Drawing for the job (mm, zero at the part's lowest x, y, z). A direction names the side the tool comes from. Coordinates: 2 decimals unless noted, no trailing zeros. Loops run counter-clockwise (first coordinate to the right, second up) from the corner with the lowest first, then second, coordinate; pieces in that order, holes last. Notation, with made-up numbers: (31.5, 75.5) - (83.5, 75.5) arc R15 cw to (83.5, 87.5) - close; hole circle Ø3 at (74, 6). An arc over 180 degrees is marked (long way). Put each result on its own line as item: value.
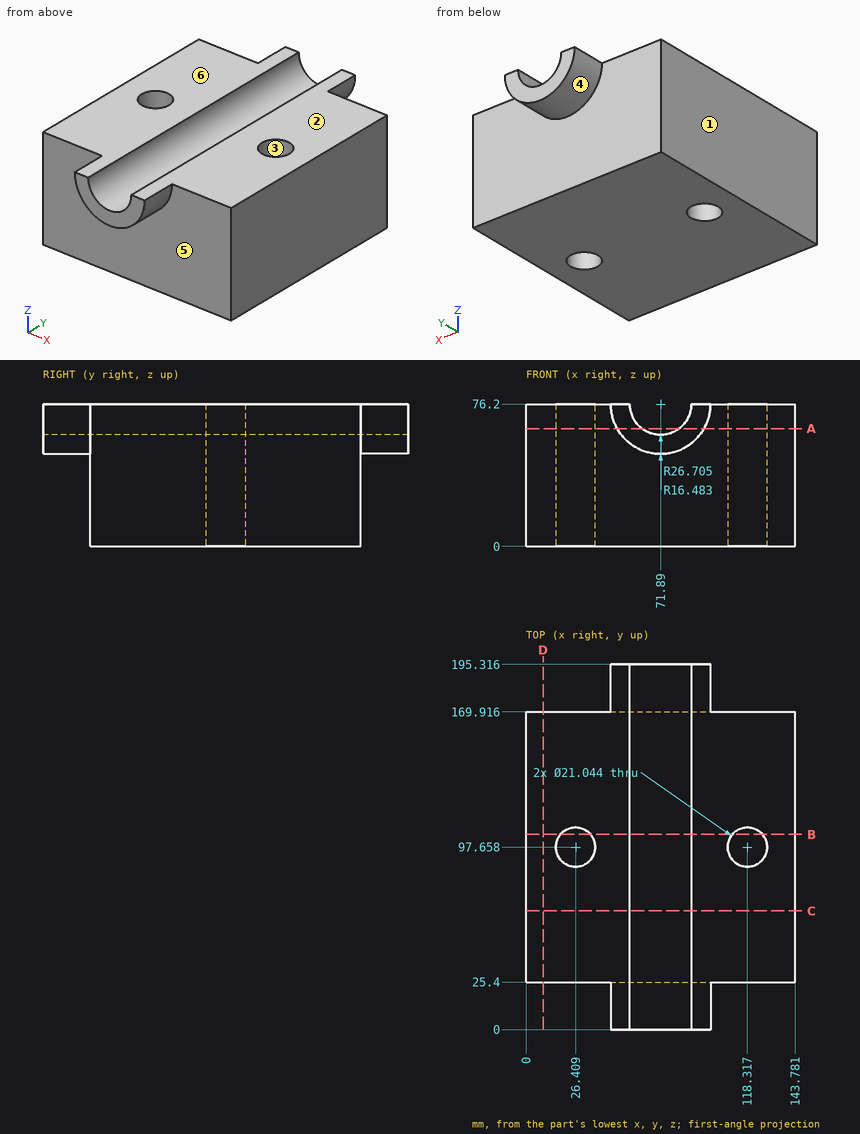
Q1. Slice it at C-C, the plane y = 63.5. Give the cut face in (x, z) (1 decimal), then the cut area to 3 significant figures.
Determined:
outline: (0, 0) - (143.8, 0) - (143.8, 76.2) - (88.4, 76.2) arc R16.5 cw to (55.4, 76.2) - (0, 76.2) - close
area: 10,500 mm2
Q2. Pin check, flat tips, straight feed: pin 1 Ø3 at (x, y) = (80.5, 169) entering from +Z; pin 2 Ø5 at (x, z) = (127.5, 46) entering from -Y; pin 3 Ø1.5 at (x, z) = (101.5, 33.5) entering from +Y. Stop position of each tip, or through.
Determined:
pin 1: z = 63.18
pin 2: y = 25.4
pin 3: y = 169.92
Q3. Slice it at D-D, the plane x = 9. Give the cut face in (y, z).
Determined:
outline: (25.4, 0) - (169.92, 0) - (169.92, 76.2) - (25.4, 76.2) - close
Q4. Wall check: L1, parallel to X at y = 91, z = 16.5 (1 decimal); L2, parallel to X at y = 93.5, z = 37 (1 decimal); L3, parallel to X at y = 151, z = 65.5 (1 decimal). Give the ranges that are in metal, low to high. Write a range as from..to.
Determined:
L1: 0..18.3, 34.6..110.2, 126.5..143.8
L2: 0..16.7, 36.1..108.7, 128..143.8
L3: 0..59.4, 84.4..143.8
Q5. Slice it at B-B, the plane y = 104.5. Give the cut face in (x, z) (1 decimal).
Determined:
outline: (0, 0) - (18.4, 0) - (18.4, 76.2) - (0, 76.2) - close; (34.4, 0) - (110.3, 0) - (110.3, 76.2) - (88.4, 76.2) arc R16.5 cw to (55.4, 76.2) - (34.4, 76.2) - close; (126.3, 0) - (143.8, 0) - (143.8, 76.2) - (126.3, 76.2) - close
Q6. Tool access for the marked faces 4, 5 and 6: list every direction of +Z, -Z, +X, -X, +Y, -Y with a clear straight run to the whole face (end or side of a thin tool).
Determined:
face 4: -Z, +Y
face 5: -Z, -Y
face 6: +Z, +X, -X, +Y, -Y
Q7. Mould opens along X. For the marked faces 1, 2 and 3 say: +X half, -X half, draft (parallel to the pull), parting line (faces both ways), or undercut.
Determined:
face 1: -X half
face 2: draft
face 3: undercut
Q8. Slice it at A-A, the plane z = 63. Give the cut face in (x, y) (1 decimal), then the cut area to 3 significant figures.
Determined:
outline: (0, 25.4) - (48.7, 25.4) - (48.7, 0) - (62, 0) - (62, 195.3) - (48.7, 195.3) - (48.7, 169.9) - (0, 169.9) - close; (81.8, 0) - (95.1, 0) - (95.1, 25.4) - (143.8, 25.4) - (143.8, 169.9) - (95.1, 169.9) - (95.1, 195.3) - (81.8, 195.3) - close; hole circle Ø21 at (26.4, 97.7); hole circle Ø21 at (118.3, 97.7)
area: 18,600 mm2
